Geometry: final body of the model. Coordinates: model frame, mm. Coordinates: 2 decimals unless noted, no trailing zeros. Loops run counter-clockwise (first coordinate to the right, second up) from the corner with the lowest first, then second, coordinate; pieces in that order, holes last. Notation, with made-up numbers: M 52.5,54 L 103.5,54 A9 cw 103.5,63 Z; hole C 44.25,3 d5. An arc over 180 degrees is marked long. Write item = value, one per line. Start each with the question number.
```python
from build123d import *

# Parameters (mm, degrees)
F0_R     = 1.5
F1_DEPTH = 2


with BuildPart() as f1:
    # F0 (on Top) → F1 (new body)
    with BuildSketch(Plane.XY):
        with BuildLine():
            ThreePointArc((-19.697627, 1), (-18.579593, 1.5), (-17.461559, 1))
            Line((-17.461559, 1), (-16.105791, 1))
            ThreePointArc((-16.105791, 1), (-15.197296, 1.218249), (-14.487079, 1.825363))
            ThreePointArc((-14.487079, 1.825363), (-13.370764, 2.775222), (-11.943263, 3.107833))
            Line((-11.943263, 3.107833), (9.535083, 2.911781))
            ThreePointArc((9.535083, 2.911781), (12.420407, 0), (9.535083, -2.911781))
            Line((9.535083, -2.911781), (-11.943263, -3.107833))
            ThreePointArc((-11.943263, -3.107833), (-13.370764, -2.775222), (-14.487079, -1.825363))
            ThreePointArc((-14.487079, -1.825363), (-15.197296, -1.218249), (-16.105791, -1))
            Line((-16.105791, -1), (-17.461559, -1))
            ThreePointArc((-17.461559, -1), (-18.579593, -1.5), (-19.697627, -1))
            Line((-19.697627, -1), (-21.850744, -1))
            ThreePointArc((-21.850744, -1), (-22.759239, -1.218249), (-23.469456, -1.825363))
            ThreePointArc((-23.469456, -1.825363), (-24.560498, -2.762335), (-25.956535, -3.107833))
            Line((-25.956535, -3.107833), (-47.215056, -3.301877))
            ThreePointArc((-47.215056, -3.301877), (-48.633493, -3.67314), (-49.706572, -4.67229))
            Line((-49.706572, -4.67229), (-51.647468, -7.672617))
            ThreePointArc((-51.647468, -7.672617), (-53.094256, -9.013578), (-55.006, -9.5))
            Line((-55.006, -9.5), (-70.66538, -9.5))
            ThreePointArc((-70.66538, -9.5), (-71.048063, -9.42388), (-71.372486, -9.207107))
            Line((-71.372486, -9.207107), (-71.7867, -8.792893))
            ThreePointArc((-71.7867, -8.792893), (-72.111123, -8.57612), (-72.493807, -8.5))
            Line((-72.493807, -8.5), (-93.829593, -8.5))
            ThreePointArc((-93.829593, -8.5), (-94.5367, -8.792893), (-94.829593, -9.5))
            Line((-94.829593, -9.5), (-94.829593, -14.497718))
            ThreePointArc((-94.829593, -14.497718), (-94.5367, -15.204825), (-93.829593, -15.497718))
            Line((-93.829593, -15.497718), (-53.964611, -15.497718))
            ThreePointArc((-53.964611, -15.497718), (-52.081116, -15.02652), (-50.64137, -13.72394))
            Line((-50.64137, -13.72394), (-47.61983, -9.213471))
            ThreePointArc((-47.61983, -9.213471), (-46.552084, -8.243011), (-45.154781, -7.883263))
            Line((-45.154781, -7.883263), (102.117442, -6.538983))
            ThreePointArc((102.117442, -6.538983), (106.230219, -7.07487), (110.039026, -8.716546))
            Line((110.039026, -8.716546), (120.015907, -14.773938))
            ThreePointArc((120.015907, -14.773938), (121.26352, -15.315064), (122.610798, -15.5))
            Line((122.610798, -15.5), (133.170407, -15.5))
            ThreePointArc((133.170407, -15.5), (133.877514, -15.207107), (134.170407, -14.5))
            Line((134.170407, -14.5), (134.170407, -9.5))
            ThreePointArc((134.170407, -9.5), (133.877514, -8.792893), (133.170407, -8.5))
            Line((133.170407, -8.5), (124.289625, -8.5))
            ThreePointArc((124.289625, -8.5), (123.211804, -8.352051), (122.213713, -7.91915))
            Line((122.213713, -7.91915), (111.986177, -1.709575))
            ThreePointArc((111.986177, -1.709575), (111.024134, 0), (111.986177, 1.709575))
            Line((111.986177, 1.709575), (122.213713, 7.91915))
            ThreePointArc((122.213713, 7.91915), (123.211804, 8.352051), (124.289625, 8.5))
            Line((124.289625, 8.5), (133.170407, 8.5))
            ThreePointArc((133.170407, 8.5), (133.877514, 8.792893), (134.170407, 9.5))
            Line((134.170407, 9.5), (134.170407, 14.5))
            ThreePointArc((134.170407, 14.5), (133.877514, 15.207107), (133.170407, 15.5))
            Line((133.170407, 15.5), (122.610798, 15.5))
            ThreePointArc((122.610798, 15.5), (121.26352, 15.315064), (120.015907, 14.773938))
            Line((120.015907, 14.773938), (110.039026, 8.716546))
            ThreePointArc((110.039026, 8.716546), (106.230219, 7.07487), (102.117442, 6.538983))
            Line((102.117442, 6.538983), (-45.154781, 7.883263))
            ThreePointArc((-45.154781, 7.883263), (-46.552084, 8.243011), (-47.61983, 9.213471))
            Line((-47.61983, 9.213471), (-50.64137, 13.72394))
            ThreePointArc((-50.64137, 13.72394), (-52.081116, 15.02652), (-53.964611, 15.497718))
            Line((-53.964611, 15.497718), (-93.829593, 15.497718))
            ThreePointArc((-93.829593, 15.497718), (-94.5367, 15.204825), (-94.829593, 14.497718))
            Line((-94.829593, 14.497718), (-94.829593, 9.5))
            ThreePointArc((-94.829593, 9.5), (-94.5367, 8.792893), (-93.829593, 8.5))
            Line((-93.829593, 8.5), (-72.493807, 8.5))
            ThreePointArc((-72.493807, 8.5), (-72.111123, 8.57612), (-71.7867, 8.792893))
            Line((-71.7867, 8.792893), (-71.372486, 9.207107))
            ThreePointArc((-71.372486, 9.207107), (-71.048063, 9.42388), (-70.66538, 9.5))
            Line((-70.66538, 9.5), (-55.006, 9.5))
            ThreePointArc((-55.006, 9.5), (-53.094256, 9.013578), (-51.647468, 7.672617))
            Line((-51.647468, 7.672617), (-49.706572, 4.67229))
            ThreePointArc((-49.706572, 4.67229), (-48.633493, 3.67314), (-47.215056, 3.301877))
            Line((-47.215056, 3.301877), (-25.956535, 3.107833))
            ThreePointArc((-25.956535, 3.107833), (-24.560498, 2.762335), (-23.469456, 1.825363))
            ThreePointArc((-23.469456, 1.825363), (-22.759239, 1.218249), (-21.850744, 1))
            Line((-21.850744, 1), (-19.697627, 1))
        make_face()
        with Locations((-91.579593, -12)):
            Circle(F0_R, mode=Mode.SUBTRACT)
        with Locations((-85.579593, -12)):
            Circle(F0_R, mode=Mode.SUBTRACT)
        with Locations((124.920407, -12)):
            Circle(F0_R, mode=Mode.SUBTRACT)
        with Locations((130.920407, -12)):
            Circle(F0_R, mode=Mode.SUBTRACT)
        with Locations((-91.579593, 12)):
            Circle(F0_R, mode=Mode.SUBTRACT)
        with Locations((-85.579593, 12)):
            Circle(F0_R, mode=Mode.SUBTRACT)
        with BuildLine():
            ThreePointArc((73.110114, 2.331478), (75.420407, 0), (73.110114, -2.331478))
            Line((73.110114, -2.331478), (30.168819, -2.72344))
            ThreePointArc((30.168819, -2.72344), (27.420407, 0), (30.168819, 2.72344))
            Line((30.168819, 2.72344), (73.110114, 2.331478))
        make_face(mode=Mode.SUBTRACT)
        with Locations((95.920407, 0)):
            Circle(F0_R, mode=Mode.SUBTRACT)
        with Locations((124.920407, 12)):
            Circle(F0_R, mode=Mode.SUBTRACT)
        with Locations((130.920407, 12)):
            Circle(F0_R, mode=Mode.SUBTRACT)
    extrude(amount=F1_DEPTH)


solid = f1.part
```
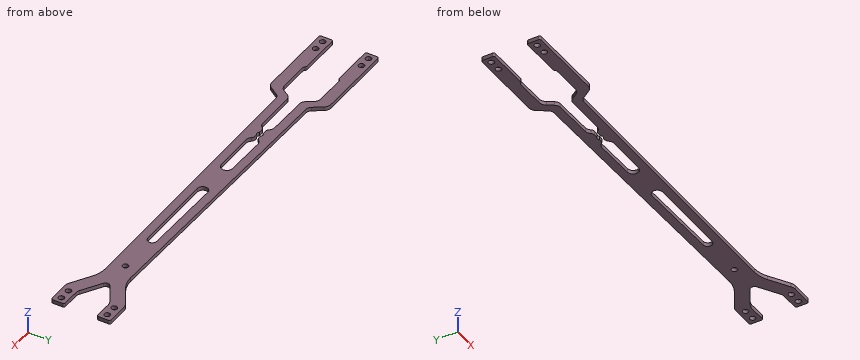
Item 1: Line query: line 1 (X direction, y = 11.5, z = 0.75); line 2 (Y direction, x = -65, z = 1.45); line 3 (Y direction, x = -75.5, z = 1.7). Output: solid intervals per line, ascending. Write a range as from..to.
Item 2: Section query A-A (x = -41.5). Return the cut outline in (y, z), plus the area to 3 significant figures.
Item 3: Section query B-B (z = 1.65). Count the separate pieces of the cut face and the enclosed holes in it, plus the area to 3 significant figures.
Item 4: Section query C-C (x = 57.5). Return the cut outline in (y, z).
Item 5: First-contact query: pin 1 (0.7 mm diameter, centred on x = -17, z = 1, fed in from -Y); pin 2 (0.6 mm diameter, centred on x = -20, z = 1, fed in from -Y); pin 3 (0.6 mm diameter, centred on x = -86, z = 1, fed in from +Y). Flat tips, straight axial feed; report the tip coordinate or a pass-through.
Verdict:
q1.line_1 = -94.83..-92.99, -90.17..-86.99, -84.17..-49.15, 114.62..123.51, 126.33..129.51, 132.33..134.17
q1.line_2 = -15.5..-9.5, 9.5..15.5
q1.line_3 = -15.5..-8.5, 8.5..15.5
q2.outline = M -7.85,0 L -3.25,0 L -3.25,2 L -7.85,2 Z; M 3.25,0 L 7.85,0 L 7.85,2 L 3.25,2 Z
q2.area = 18.4 mm2
q3.separate_pieces = 1
q3.enclosed_holes = 10
q3.area = 2,640 mm2
q4.outline = M -6.95,0 L -2.47,0 L -2.47,2 L -6.95,2 Z; M 2.47,0 L 6.95,0 L 6.95,2 L 2.47,2 Z
q5.pin_1 = -7.63
q5.pin_2 = -7.66
q5.pin_3 = 15.5
